Here's how the part is built. I have some questions about the finished solid (model axes, mm). Give positions to 0.01 mm unless a question says otherwise; leave off trailing zeros. Write each loop counter-clockwise with the first axis right and the second up, starting at its lowest first coordinate (ties: lowest second). Pieces come first, ordered by that corner, then holes. Notation, with made-up numbers: (88.25, -24.5) - (146.25, -24.5) arc R35 ccw to (146.25, 8.5) - close; hole circle Ø1 at (-0.75, -16.5). An arc over 180 degrees is marked (long way). Use one line per item in the form item = value. Start each with the question number.
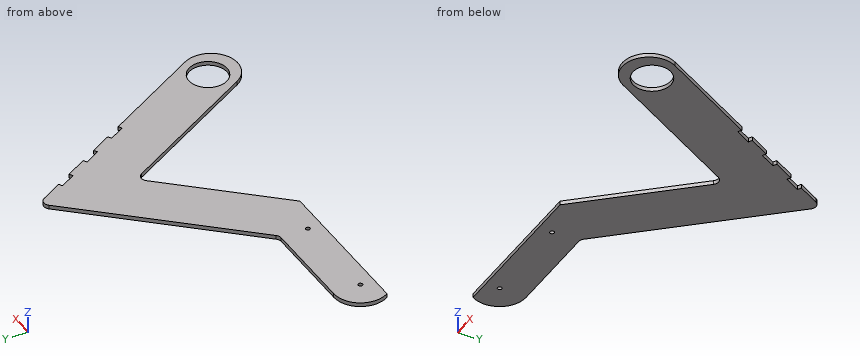
from build123d import *

# Parameters (mm, degrees)
CROQUIS1_R              = 1.58
CROQUIS1_R_2            = 14.25
SALIENTE_EXTRUIR1_DEPTH = 3
CROQUIS3_W              = 3
CROQUIS3_H              = 13.002457907
CROQUIS3_H_2            = 13.048194377
CROQUIS3_H_3            = 13.048194378
CORTAR_EXTRUIR1_DEPTH   = 3
CROQUIS4_W              = 144.23908533
CROQUIS4_H              = 10
CORTAR_EXTRUIR2_DEPTH   = 10


with BuildPart() as part:
    # Croquis1 → Saliente-Extruir1 (new body)
    with BuildSketch(Plane.XY):
        with BuildLine():
            Line((-135.811178416, 31.660861846), (-65.873242367, 31.660861846))
            ThreePointArc((-65.873242367, 31.660861846), (-63.837291884, 32.094144685), (-62.154198363, 33.318899594))
            Line((-62.154198363, 33.318899594), (39.488020824, 146.429658271))
            ThreePointArc((39.488020824, 146.429658271), (43.775922453, 148.055230719), (47.585333219, 145.502393908))
            Line((47.585333219, 145.502393908), (132.043103592, -7.634273033))
            ThreePointArc((132.043103592, -7.634273033), (124.188821584, -34.806138154), (97.016956463, -26.951856146))
            Line((97.016956463, -26.951856146), (39.731279169, 76.917067288))
            ThreePointArc((39.731279169, 76.917067288), (35.921868403, 79.4699041), (31.633966774, 77.844331652))
            Line((31.633966774, 77.844331652), (-44.321252629, -6.681100406))
            ThreePointArc((-44.321252629, -6.681100406), (-46.00434615, -7.905855315), (-48.040296633, -8.339138154))
            Line((-48.040296633, -8.339138154), (-135.811178416, -8.339138154))
            ThreePointArc((-135.811178416, -8.339138154), (-155.811178416, 11.660861846), (-135.811178416, 31.660861846))
        make_face()
        with Locations((-135.811178416, 11.660861846)):
            Circle(CROQUIS1_R, mode=Mode.SUBTRACT)
        with Locations((-65.81121578, 11.5885363)):
            Circle(CROQUIS1_R, mode=Mode.SUBTRACT)
        with Locations((112.738617641, -14.044921514)):
            Circle(CROQUIS1_R_2, mode=Mode.SUBTRACT)
    extrude(amount=SALIENTE_EXTRUIR1_DEPTH)

    # Croquis3 → Cortar-Extruir1 (cut)
    with BuildSketch(Plane(origin=(98.018165522, 54.058873563, 0), x_dir=(0, 0, -1), z_dir=(0.875653678217041, 0.4829395778200074, 0))):
        with Locations((-1.5, 79.927636726)):
            Rectangle(CROQUIS3_W, CROQUIS3_H)
        with Locations((-1.5, 49.42886568)):
            Rectangle(CROQUIS3_W, CROQUIS3_H_2)
        with Locations((-1.5, 18.952962868)):
            Rectangle(CROQUIS3_W, CROQUIS3_H_3)
    extrude(amount=-CORTAR_EXTRUIR1_DEPTH, mode=Mode.SUBTRACT)

    # Croquis4 → Cortar-Extruir2 (cut)
    with BuildSketch(Plane.XY.offset(3)):
        with Locations((-102.474853033, -3.605700694)):
            Rectangle(CROQUIS4_W, CROQUIS4_H)
    extrude(amount=-CORTAR_EXTRUIR2_DEPTH, mode=Mode.SUBTRACT)


solid = part.part
1. Please list where these lines run through material, in increasing order: line 1 (Y direction, x = -112, z = 0.5); line 2 (X direction, y = -20.5, z = 2.6); line 3 (X direction, y = -4, z = 1.4).
2. I want a section at D-D, the plane x = -130. List the corners of the cut face in (y, z) for me, then the cut area to 3 significant figures.
3. For P1, Ø3, axis at x = 71, y = 76, coming from the -Z side; P2, Ø0.9, axis at x = -87, z = 1, coming from the +Y side; P3, Ø1.5, axis at y = 58.5, z = 2.5, coming from the +X side; P4, Ø0.9, axis at x = -95, z = 1.5, coming from the -Y side, each with a flat end and sliding along its axis, tell me the tip position at first contact or that it passes through.
4. I want a section at A-A, the plane x = 107.5. List the corners of the cut face in (y, z) for me.
5. I want a section at B-B, the plane y = 46. List the corners of the cut face in (x, z) for me.
6. I want a section at C-C, the plane z = 2.55. List the corners of the cut face in (x, y) for me, then the cut area to 3 significant figures.
Result sheet:
q1.line_1 = 1.39 to 31.66
q1.line_2 = 93.46 to 100.03, 125.44 to 134.27
q1.line_3 = 84.36 to 102.63, 122.85 to 130.04
q2.outline = (1.39, 0) - (31.66, 0) - (31.66, 3) - (1.39, 3) - close
q2.area = 90.8 mm2
q3.P1 = 0
q3.P2 = 31.66
q3.P3 = 95.98
q3.P4 = 1.39
q4.outline = (-36.02, 0) - (-27.3, 0) - (-27.3, 3) - (-36.02, 3) - close; (-0.79, 0) - (36.87, 0) - (36.87, 3) - (-0.79, 3) - close
q5.outline = (-50.76, 0) - (3.02, 0) - (3.02, 3) - (-50.76, 3) - close; (56.78, 0) - (102.46, 0) - (102.46, 3) - (56.78, 3) - close
q6.outline = (-152.98, 1.39) - (-37.06, 1.39) - (31.63, 77.84) arc R5 cw to (39.73, 76.92) - (97.02, -26.95) arc R20 ccw to (132.04, -7.63) - (92.02, 64.94) - (89.39, 63.49) - (83.09, 74.92) - (85.71, 76.37) - (77.3, 91.63) - (74.67, 90.18) - (68.37, 101.61) - (71, 103.05) - (62.56, 118.35) - (59.93, 116.91) - (53.65, 128.29) - (56.28, 129.74) - (47.59, 145.5) arc R5 ccw to (39.49, 146.43) - (-62.15, 33.32) arc R5 cw to (-65.87, 31.66) - (-135.81, 31.66) arc R20 ccw to start; hole circle Ø3.16 at (-135.81, 11.66); hole circle Ø3.16 at (-65.81, 11.59); hole circle Ø28.5 at (112.74, -14.04)
q6.area = 14,500 mm2
